from build123d import *

# Parameters (mm, degrees)
F0_W      = 1524
F0_H      = 1016
F1_DEPTH  = 1016
F2_W      = 1016
F2_H      = 762
F3_DEPTH  = 254
F5_DEPTH  = 762
F6_W      = 508
F6_H      = 254
F7_DEPTH  = 254
F8_W      = 508
F8_H      = 508
F9_DEPTH  = 254
F11_DEPTH = 254
F12_R     = 254
F13_DEPTH = 254
F15_DEPTH = 254


with BuildPart() as f1:
    # F0 (on Front) → F1 (new body)
    with BuildSketch(Plane.XZ):
        with Locations((762, 508)):
            Rectangle(F0_W, F0_H)
    extrude(amount=F1_DEPTH)

    # F2 (on face) → F3 (cut)
    with BuildSketch(Plane.XZ.offset(1016)):
        with Locations((1016, 635)):
            Rectangle(F2_W, F2_H)
    extrude(amount=-F3_DEPTH, mode=Mode.SUBTRACT)

    # F4 (on face) → F5 (cut)
    with BuildSketch(Plane.XY.offset(1016)):
        Polygon((0, -762), (508, -762), (1524, -762), (1524, -254), (0, -254), align=None)
    extrude(amount=-F5_DEPTH, mode=Mode.SUBTRACT)

    # F6 (on face) → F7 (cut)
    with BuildSketch(Plane.XZ.offset(1016)):
        with Locations((254, 889)):
            Rectangle(F6_W, F6_H)
    extrude(amount=-F7_DEPTH, mode=Mode.SUBTRACT)

    # F8 (on face) → F9 (cut)
    with BuildSketch(Plane.XZ.offset(254)):
        with Locations((254, 762)):
            Rectangle(F8_W, F8_H)
    extrude(amount=-F9_DEPTH, mode=Mode.SUBTRACT)

    # F10 (on face) → F11 (cut)
    with BuildSketch(Plane.XZ.offset(254)):
        with BuildLine():
            Line((1524, 1016), (1016, 1016))
            ThreePointArc((1016, 1016), (1375.210245, 867.210245), (1524, 508))
            Line((1524, 508), (1524, 1016))
        make_face()
        with BuildLine():
            Line((508, 1016), (508, 508))
            ThreePointArc((508, 508), (656.789755, 867.210245), (1016, 1016))
            Line((1016, 1016), (508, 1016))
        make_face()
    extrude(amount=-F11_DEPTH, mode=Mode.SUBTRACT)

    # F12 (on face) → F13 (cut)
    with BuildSketch(Plane.XZ.offset(254)):
        with Locations((988.703072, 493.149191)):
            Circle(F12_R)
    extrude(amount=-F13_DEPTH, mode=Mode.SUBTRACT)

    # F14 (on face) → F15 (cut)
    with BuildSketch(Plane.XZ.offset(1016)):
        with BuildLine():
            Line((508, 762), (275.637895, 762))
            ThreePointArc((275.637895, 762), (284.796354, 509.020591), (508, 389.5945))
            Line((508, 389.5945), (508, 762))
        make_face()
    extrude(amount=-F15_DEPTH, mode=Mode.SUBTRACT)


solid = f1.part
Build history of the part. All positions in model axes, mm. A direction names the side the tool comes from. Round coordinates to 2 decimals unless told otherwise and drop trailing zeros. Write each loop counter-clockwise with the first axis right and the second up, starting at its lowest first coordinate (ties: lowest second). Pieces come first, ordered by that corner, then holes. Notation, with made-up numbers: M -7,-33 L 42,-33 A9 cw 42,-22 Z; hole C -34.5,13 d8. An arc over 180 degrees is marked long. Answer in a Markdown table with one row per item.
1. Probe L1, parallel to Z at x = 1294, y = -636.5; L2, parallel to Y at x = 962, z = 819; L3, parallel to X at y = -173, z = 474. List the from-to ranges inside material, lowest first. Write a range as [from, to].
Geometry check:
| item | result |
|---|---|
| L1 | [0, 254] |
| L2 | [-254, 0] |
| L3 | [0, 735.43], [1241.98, 1524] |
2. Saw through at C-C (x = 211.5). List the corners of the cut face in (y, z).
Geometry check:
| item | result |
|---|---|
| outline | M -1016,0 L 0,0 L 0,508 L -254,508 L -254,254 L -762,254 L -762,762 L -1016,762 Z |
3. Flat gauge pins, fed straight in: P1, Ø12, axis at x = 987.5, z = 248.5, coming from the +Y side; P2, Ø1, axis at x = 1343.5, z = 792, coming from the -Y side; P3, Ø2, axis at x = 538.5, y = -199, coming from the -Z side. Where does each tip first touch, or does it go through?
Geometry check:
| item | result |
|---|---|
| P1 | y = -254 |
| P2 | y = -254 |
| P3 | z = 0 |
4. Saw through at A-A (z = 599.5). List the corners of the cut face in (x, y), and give its area (3 significant figures).
Geometry check:
| item | result |
|---|---|
| outline | M 0,-1016 L 250.13,-1016 L 250.13,-762 L 0,-762 Z; M 516.31,-254 L 758.04,-254 L 758.04,0 L 516.31,0 Z; M 1219.37,-254 L 1515.69,-254 L 1515.69,0 L 1219.37,0 Z |
| area | 200,000 mm2 |
5. Saw through at D-D (y = -662.5). List the corners of the cut face in (x, z), and give its area (3 significant figures).
Geometry check:
| item | result |
|---|---|
| outline | M 0,0 L 1524,0 L 1524,254 L 0,254 Z |
| area | 387,000 mm2 |
6. Mould opens along Y. For faces 4 (the face through (582, -1016, 217)), 5 (the face through (773, -254, 640)), 6 (the face through (250, -129, 508)), 7 (the face through (751, -630, 254)) say: +Y half, -Y half, draft (parallel to the pull), parting line (faces both ways), or undercut.
Geometry check:
| item | result |
|---|---|
| face 4 | -Y half |
| face 5 | undercut |
| face 6 | draft |
| face 7 | undercut |
7. Saw through at B-B (x = 872.5). List the corners of the cut face in (y, z).
Geometry check:
| item | result |
|---|---|
| outline | M -1016,0 L 0,0 L 0,267.29 L -254,267.29 L -254,254 L -1016,254 Z; M -254,719.01 L 0,719.01 L 0,995.31 L -254,995.31 Z |
8. Which spindle directions (+Z, -Z, +X, -X, +Y, -Y) get a long thin tool onto all of the face, cutting with end or side? Do faces 1 (the face through (194, -762, 455)), 2 (the face through (136, -891, 762)), 3 (the face through (508, -891, 321)). Say none if no direction does.
Geometry check:
| item | result |
|---|---|
| face 1 | +Z, +X, -X |
| face 2 | +Z, +X, -X, +Y, -Y |
| face 3 | +Z, +X, -Y |
